```python
from build123d import *

# Parameters (mm, degrees)
F0_W           = 27
F0_H           = 225
F1_DEPTH       = 6.35
F2_R           = 6.35
F4_D           = 5.5
F4_CBORE_D     = 8.5
F4_CBORE_DEPTH = 3.5
F6_D           = 3.3


with BuildPart() as f1:
    # F0 (on Front) → F1 (new body)
    with BuildSketch(Plane.XZ):
        Rectangle(F0_W, F0_H)
    extrude(amount=F1_DEPTH)

    # F2
    f2_edges = [f1.edges().sort_by_distance(p)[0] for p in [
        (13.5, -3.175, 112.5),
        (-13.5, -3.175, 112.5),
        (13.5, -3.175, -112.5),
        (-13.5, -3.175, -112.5),
    ]]
    fillet(f2_edges, radius=F2_R)

    # F4 (through all)
    with Locations(Plane.XZ.offset(6.35)):
        with Locations((-8, 26), (8, 26), (-8, -26), (8, -26)):
            CounterBoreHole(F4_D / 2, F4_CBORE_D / 2, F4_CBORE_DEPTH)

    # F6 (through all)
    with Locations(Plane(origin=(0, 0, 0), x_dir=(-1, 0, 0), z_dir=(0, 1, 0))):
        with Locations((0, 101.6), (0, -101.6)):
            Hole(F6_D / 2)


solid = f1.part
```
Source: CAD feature listing. Evaluate the final solid. Frame: model axes, mm. A direction names the side the tool comes from. Coordinates: 2 decimals unless noted, no trailing zeros. Write each loop counter-clockwise with the first axis right and the second up, starting at its lowest first coordinate (ties: lowest second). Pieces come first, ordered by that corner, then holes. Notation, with made-up numbers: (-10.75, 73) -> (40.25, 73) arc R20 ccw to (40.25, 91) -> close; hole circle Ø5 at (-15.75, 54). An arc over 180 degrees is marked (long way). Return JSON: item names as keys, results as strings. Group by question number.
1) Ray query, line 1 along Z through (x, y) = (0, -3.75); line 2 along Z through (x, y) = (5.5, -1.5); line 3 along X through (y, z) = (-3.25, -29.5). Return the intervals inside material, ascending.
2) Section query B-B, the plane y = -1. Return loops of the section in (x, z), plus the area to 3 significant figures.
3) Contact query for flat-ended pins moving along their axis: P1, Ø3.5, axis at x = -8, z = 26, coming from the +Y side; P2, Ø4, axis at x = -6.5, z = -24.5, coming from the -Y side. Output: stop coordinate, or through.
4) Mould query, pull axis Z, two halves, no side actions, for faces 3 (the face through (-11.37, -4.62, -28.59)), 4 (the face through (11.69, -3.22, 110.59)), 5 (the face through (13.5, -3, -1)), 6 (the face through (0, -3, -112.5)). Classes: +Z half, -Z half, draft (parallel to the pull), parting line (faces both ways), or undercut.
5) Set-up query: faces 1 (the face through (-8.553, -4.624, 30.214)), 2 (the face through (8.358, -1.405, -23.273)). Return all of +Z, -Z, +X, -X, +Y, -Y with unobstructed straight access to the full face (end or side cutting, diameter ignored); none if empty.
6) Section query A-A, the plane z = 26. Return loops of the section in (x, y).
From the geometry:
{
 "1": {"line 1": "-112.5 to -103.25, -99.95 to 99.95, 103.25 to 112.5", "line 2": "-112.5 to -27.15, -24.85 to 24.85, 27.15 to 112.5", "line 3": "-13.5 to -10.41, -5.59 to 5.59, 10.41 to 13.5"},
 "2": {"outline": "(-13.5, -106.15) arc R6.35 ccw to (-7.15, -112.5) -> (7.15, -112.5) arc R6.35 ccw to (13.5, -106.15) -> (13.5, 106.15) arc R6.35 ccw to (7.15, 112.5) -> (-7.15, 112.5) arc R6.35 ccw to (-13.5, 106.15) -> close; hole circle Ø5.5 at (-8, -26); hole circle Ø5.5 at (-8, 26); hole circle Ø3.3 at (0, -101.6); hole circle Ø3.3 at (0, 101.6); hole circle Ø5.5 at (8, -26); hole circle Ø5.5 at (8, 26)", "area": "5,930 mm²"},
 "3": {"P1": "through", "P2": "y = -2.85"},
 "4": {"face 3": "undercut", "face 4": "+Z half", "face 5": "draft", "face 6": "-Z half"},
 "5": {"face 1": "-Y", "face 2": "+Y, -Y"},
 "6": {"outline": "(-13.5, -6.35) -> (-12.25, -6.35) -> (-12.25, -2.85) -> (-10.75, -2.85) -> (-10.75, 0) -> (-13.5, 0) -> close; (-5.25, -2.85) -> (-3.75, -2.85) -> (-3.75, -6.35) -> (3.75, -6.35) -> (3.75, -2.85) -> (5.25, -2.85) -> (5.25, 0) -> (-5.25, 0) -> close; (10.75, -2.85) -> (12.25, -2.85) -> (12.25, -6.35) -> (13.5, -6.35) -> (13.5, 0) -> (10.75, 0) -> close"}
}
